Input: part model. Units: mm. Frame: model coordinates. Give positions to 0.01 mm unless a question says otherwise; leave off trailing zeros. Write each loop counter-clockwise with the first axis right and the second up, starting at its lowest first coordinate (ties: lowest second). Pieces come first, ordered by that corner, then holes. Notation, with made-up numbers: (-28.75, 17) - (21.25, 17) arc R20 cw to (21.25, 22) - close; hole circle Ø6 at (-13, -30). An arc over 180 degrees is marked (long way). Use a Markdown table: item, result. Add a question column.
1. Section query B-B, the plane y = 0.3. Return loops of the section in (x, z) (3 decimals).
2. Section query A-A, the plane z = 41.5. Return loops of the section in (x, y).
3. Pin query (flat end, axial travel): pin 1 (1.5 mm diameter, centred on x = 31.5, z = -34, fed in from -Y). Return the tip coordinate at first contact, or that it passes through.
4. Material intervals for probe 1 along Z at (x, y) = (-56, 0.4) (3 decimals); probe 2 along X at (y, z) = (0.4, -38), sorted ascending.
```python
from build123d import *

# Parameters (mm, degrees)
SKETCH1_W           = 127
SKETCH1_H           = 101.6
BOSS_EXTRUDE1_DEPTH = 1.27
CUT_EXTRUDE1_REACH  = 83.33
SKETCH2_W           = 6.35
SKETCH2_H           = 9.525


with BuildPart() as part:
    # Sketch1 → Boss-Extrude1 (new body)
    with BuildSketch(Plane(origin=(0, 0, 0), x_dir=(1, 0, 0), z_dir=(0, 1, 0))):
        Rectangle(SKETCH1_W, SKETCH1_H)
    extrude(amount=BOSS_EXTRUDE1_DEPTH)

    # Sketch2 → Cut-Extrude1 (cut, up to next)
    with BuildSketch(Plane(origin=(0, 1.27, 0), x_dir=(1, 0, 0), z_dir=(0, 1, 0)), mode=Mode.PRIVATE) as cut_extrude1_sk1:
        with Locations((-56.515, 42.2275)):
            Rectangle(SKETCH2_W, SKETCH2_H)
    cut_extrude1_tool1 = extrude(cut_extrude1_sk1.sketch, amount=-CUT_EXTRUDE1_REACH, mode=Mode.PRIVATE) & part.part
    # Sketch2 → Cut-Extrude1 (cut, up to next)
    with BuildSketch(Plane(origin=(0, 1.27, 0), x_dir=(1, 0, 0), z_dir=(0, 1, 0)), mode=Mode.PRIVATE) as cut_extrude1_sk2:
        with Locations((56.515, 42.2275)):
            Rectangle(SKETCH2_W, SKETCH2_H)
    cut_extrude1_tool2 = extrude(cut_extrude1_sk2.sketch, amount=-CUT_EXTRUDE1_REACH, mode=Mode.PRIVATE) & part.part
    # Sketch2 → Cut-Extrude1 (cut, up to next)
    with BuildSketch(Plane(origin=(0, 1.27, 0), x_dir=(1, 0, 0), z_dir=(0, 1, 0)), mode=Mode.PRIVATE) as cut_extrude1_sk3:
        with Locations((56.515, -42.2275)):
            Rectangle(SKETCH2_W, SKETCH2_H)
    cut_extrude1_tool3 = extrude(cut_extrude1_sk3.sketch, amount=-CUT_EXTRUDE1_REACH, mode=Mode.PRIVATE) & part.part
    # Sketch2 → Cut-Extrude1 (cut, up to next)
    with BuildSketch(Plane(origin=(0, 1.27, 0), x_dir=(1, 0, 0), z_dir=(0, 1, 0)), mode=Mode.PRIVATE) as cut_extrude1_sk4:
        with Locations((-56.515, -42.2275)):
            Rectangle(SKETCH2_W, SKETCH2_H)
    cut_extrude1_tool4 = extrude(cut_extrude1_sk4.sketch, amount=-CUT_EXTRUDE1_REACH, mode=Mode.PRIVATE) & part.part
    add(cut_extrude1_tool1.solids().sort_by_distance((-56.515, 1.27, -42.2275))[0], mode=Mode.SUBTRACT)
    add(cut_extrude1_tool2.solids().sort_by_distance((56.515, 1.27, -42.2275))[0], mode=Mode.SUBTRACT)
    add(cut_extrude1_tool3.solids().sort_by_distance((56.515, 1.27, 42.2275))[0], mode=Mode.SUBTRACT)
    add(cut_extrude1_tool4.solids().sort_by_distance((-56.515, 1.27, 42.2275))[0], mode=Mode.SUBTRACT)


solid = part.part
```
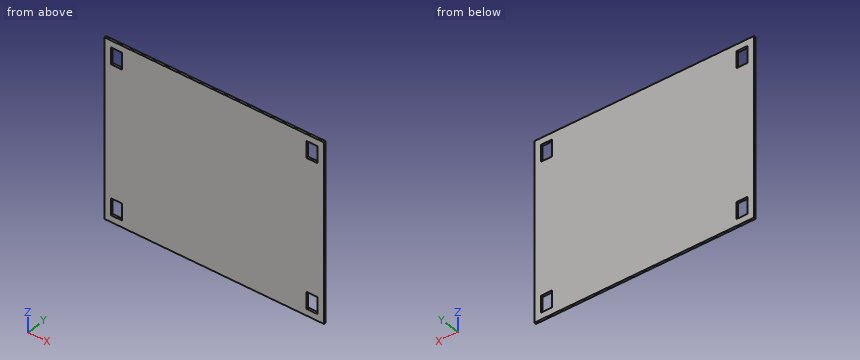
Result sheet:
| question | item | result |
|---|---|---|
| 1 | outline | (-63.5, -50.8) - (63.5, -50.8) - (63.5, 50.8) - (-63.5, 50.8) - close; hole (-59.69, -46.99) - (-53.34, -46.99) - (-53.34, -37.465) - (-59.69, -37.465) - close; hole (-59.69, 37.465) - (-53.34, 37.465) - (-53.34, 46.99) - (-59.69, 46.99) - close; hole (53.34, -46.99) - (59.69, -46.99) - (59.69, -37.465) - (53.34, -37.465) - close; hole (53.34, 37.465) - (59.69, 37.465) - (59.69, 46.99) - (53.34, 46.99) - close |
| 2 | outline | (-63.5, 0) - (-59.69, 0) - (-59.69, 1.27) - (-63.5, 1.27) - close; (-53.34, 0) - (53.34, 0) - (53.34, 1.27) - (-53.34, 1.27) - close; (59.69, 0) - (63.5, 0) - (63.5, 1.27) - (59.69, 1.27) - close |
| 3 | pin 1 | stops at y = 0 |
| 4 | probe 1 | z = -50.8 to -46.99, -37.465 to 37.465, 46.99 to 50.8 |
| 4 | probe 2 | x = -63.5 to -59.69, -53.34 to 53.34, 59.69 to 63.5 |
